Source: CAD feature listing. Evaluate the final solid. Frame: model axes, mm. A direction names the side the tool comes from. Coordinates: 2 decimals unless noted, no trailing zeros. Order: outer loops, then holes, each group sorted by start corner. A loop starts at its lowest first (then second) coordinate and runs counter-clockwise, first axis right, second up. Notation, with made-up numbers: (67, 20.5) - (113, 20.5) arc R16 cw to (113, 40.5) - close; hole circle Ø3 at (29.5, 12). An arc over 180 degrees is marked (long way). One line per question, with ' | ' between items. Start each with the question number.
(1) Contact query for flat-ended pins moving along their axis: P1, Ø0.9, axis at x = 11.5, z = 1.5, coming from the +Y side; P2, Ø0.9, axis at y = 293, z = 2, coming from the -X side; P3, Ø1.5, axis at x = 27, z = 2, coming from the +Y side; P4, Ø0.9, axis at x = 12, z = 1.5, coming from the -Y side. Output: stop coordinate, or through.
(2) Section B-B (y = 291). Return the cut outline in (x, z).
(3) Section C-C (z = 0.45). Return the cut outline in (x, y), then the cut area to 3 significant figures.
(4) Section A-A (x = 13.25). Return the cut outline in (y, z), then the cut area to 3 significant figures.
(5) Access query for faces 5 (the flat face through (19, 287.606, 1)), 6 (the flat face through (21, 293.606, 1)), 7 (the flat face through (28, 295.606, 1)). Directions: +Z, -Z, +X, -X, +Y, -Y. A direction counts if a zero-diameter tool reaches every point of the face in a straight line with its end or side. Return the directions, or none.
(6) Section D-D (x = 28). Return the cut outline in (y, z).
(7) Line query: line 1 along Y through (x, z) = (20, 1.5); line 2 along X through (y, z) = (293.5, 1.75); line 3 along X through (y, z) = (291.25, 2). Output: solid intervals per line, ascending.
(8) Draft query along X for faces 1 (the flat face through (32.282, 292, 1)), 2 (the cylindrical face through (7.783, 292.205, 1.479)), 3 (the flat face through (19.782, 292, 1)), 4 (the flat face through (28, 288.606, 1)). Return one class per face: +X half, -X half, draft (parallel to the pull), parting line (faces both ways), or undercut.
from build123d import *

# Parameters (mm, degrees)
MODEL_W                 = 3
MODEL_H                 = 3
SALIENTE_EXTRUIR2_DEPTH = 3


with BuildPart() as part:
    # Model → Saliente-Extruir2 (new body)
    with BuildSketch(Plane.XY):
        with BuildLine():
            Line((25.281533596, 296.606231861), (12.281533596, 296.606231861))
            ThreePointArc((12.281533596, 296.606231861), (7.781533596, 292.106231861), (12.281533596, 287.606231861))
            Line((12.281533596, 287.606231861), (25.281533596, 287.606231861))
            ThreePointArc((25.281533596, 287.606231861), (25.635086987, 287.752678471), (25.781533596, 288.106231861))
            Line((25.781533596, 288.106231861), (25.781533596, 288.606231861))
            Line((25.781533596, 288.606231861), (30.781533596, 288.606231861))
            ThreePointArc((30.781533596, 288.606231861), (31.842193768, 289.045571689), (32.281533596, 290.106231861))
            Line((32.281533596, 290.106231861), (32.281533596, 294.106231861))
            ThreePointArc((32.281533596, 294.106231861), (31.842193768, 295.166892033), (30.781533596, 295.606231861))
            Line((30.781533596, 295.606231861), (25.781533596, 295.606231861))
            Line((25.781533596, 295.606231861), (25.781533596, 296.106231861))
            ThreePointArc((25.781533596, 296.106231861), (25.635086987, 296.459785252), (25.281533596, 296.606231861))
        make_face()
        with Locations((12.281533596, 292.106231861)):
            Rectangle(MODEL_W, MODEL_H, mode=Mode.SUBTRACT)
        with Locations((21.281533596, 292.106231861)):
            Rectangle(MODEL_W, MODEL_H, mode=Mode.SUBTRACT)
    extrude(amount=SALIENTE_EXTRUIR2_DEPTH)


solid = part.part
Response values:
1) P1: stops at y = 296.59 | P2: stops at x = 7.8 | P3: stops at y = 295.61 | P4: stops at y = 287.61
2) outline: (7.92, 0) - (10.78, 0) - (10.78, 3) - (7.92, 3) - close; (13.78, 0) - (19.78, 0) - (19.78, 3) - (13.78, 3) - close; (22.78, 0) - (32.28, 0) - (32.28, 3) - (22.78, 3) - close
3) outline: (12.28, 287.61) - (25.28, 287.61) arc R0.5 ccw to (25.78, 288.11) - (25.78, 288.61) - (30.78, 288.61) arc R1.5 ccw to (32.28, 290.11) - (32.28, 294.11) arc R1.5 ccw to (30.78, 295.61) - (25.78, 295.61) - (25.78, 296.11) arc R0.5 ccw to (25.28, 296.61) - (12.28, 296.61) arc R4.5 ccw to start; hole (10.78, 290.61) - (13.78, 290.61) - (13.78, 293.61) - (10.78, 293.61) - close; hole (19.78, 290.61) - (22.78, 290.61) - (22.78, 293.61) - (19.78, 293.61) - close | area: 180 mm²
4) outline: (287.61, 0) - (290.61, 0) - (290.61, 3) - (287.61, 3) - close; (293.61, 0) - (296.61, 0) - (296.61, 3) - (293.61, 3) - close | area: 18.0 mm²
5) face 5: +Z, -Z, +X, -X, -Y | face 6: +Z, -Z | face 7: +Z, -Z, +X, +Y
6) outline: (288.61, 0) - (295.61, 0) - (295.61, 3) - (288.61, 3) - close
7) line 1: y = 287.61 to 290.61, 293.61 to 296.61 | line 2: x = 8 to 10.78, 13.78 to 19.78, 22.78 to 32.28 | line 3: x = 7.86 to 10.78, 13.78 to 19.78, 22.78 to 32.28
8) face 1: +X half | face 2: -X half | face 3: undercut | face 4: draft
